Verification items for the finished model (mm, model axes). Face numbers are marked on the shaded views. A direction names the side the tool comes from. Round coordinates to 2 decimals unless told otherwise and drop trailing zeros. Write each loop counter-clockwise with the first axis right and the second up, starting at its lowest first coordinate (ties: lowest second). Pieces come first, ordered by that corner, then holes.
from build123d import *

# Parameters (mm, degrees)
BOSS_EXTRUDE1_DEPTH = 15.85
SHELL1_T            = -1.5


with BuildPart() as part:
    # Sketch1 → Boss-Extrude1 (new body)
    with BuildSketch(Plane(origin=(0, 0, 0), x_dir=(0, 0, -1), z_dir=(1, 0, 0))):
        with BuildLine():
            Line((0, 9.5), (0, 0))
            Line((0, 0), (-7.8, 0))
            ThreePointArc((-7.8, 0), (-5.600175557, 6.145933615), (0, 9.5))
        make_face()
    extrude(amount=-BOSS_EXTRUDE1_DEPTH)

    # Shell1
    shell1_openings = [part.faces().sort_by_distance(p)[0] for p in [
        (-7.925, 0, 3.9),
    ]]
    offset(amount=SHELL1_T, openings=shell1_openings, kind=Kind.INTERSECTION)


solid = part.part
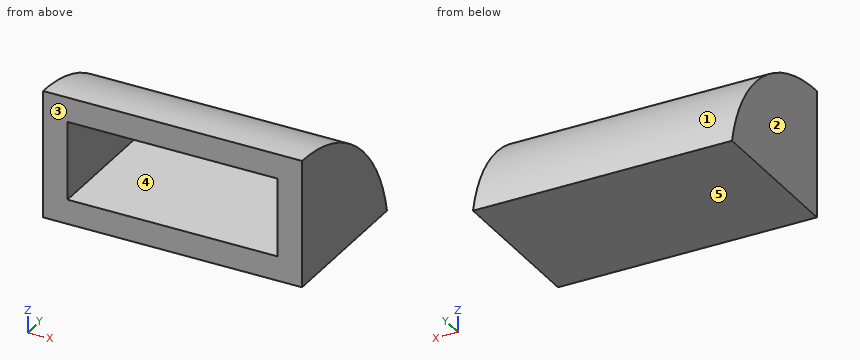
Q1. Sectioned sample at B-B (x = -2.75). Enter the section's corners in (y, z), plus the area to 3 significant figures.
Recorded:
outline: (0, 0) - (9.5, 0) arc R9.69 ccw to (0, 7.8) - (0, 6.3) arc R8.19 cw to (7.45, 1.5) - (0, 1.5) - close
area: 29.8 mm2
Q2. Tool access check on the marked faces 4 and 5. Record the directions out of +Z, -Z, +X, -X, +Y, -Y that give a thin tool (end or side, any length) a straight path to the whole face; none if there is none.
Recorded:
face 4: -Y
face 5: -Z, +X, -X, +Y, -Y
Q3. Sectioned sample at D-D (y = 1.5). Enter the section's corners in (x, z).
Recorded:
outline: (-15.85, 0) - (0, 0) - (0, 7.68) - (-15.85, 7.68) - close; hole (-14.35, 1.5) - (-1.5, 1.5) - (-1.5, 6.16) - (-14.35, 6.16) - close
Q4. Sectioned sample at C-C (z = 5). Enter the section's corners in (x, y).
Recorded:
outline: (-15.85, 0) - (-14.35, 0) - (-14.35, 4.43) - (-1.5, 4.43) - (-1.5, 0) - (0, 0) - (0, 6.81) - (-15.85, 6.81) - close
Q5. Material ranges on line 1 along X through (y, z) = (5.25, 2.25); line 2 along Z through (x, y) = (-7.75, 5.25); line 3 along Z through (x, y) = (-10.25, 3.25), recorded low to high.
Recorded:
line 1: x = -15.85 to -14.35, -1.5 to 0
line 2: z = 0 to 1.5, 4.39 to 6.25
line 3: z = 0 to 1.5, 5.63 to 7.24
Q6. Release check for a two-part mould opening along Y. For the marked faces 1, 2 and 3 record: released by +Y, released by -Y, zero draft, split by the parting line, or undercut.
Recorded:
face 1: released by +Y
face 2: zero draft
face 3: released by -Y
Q7. Sectioned sample at A-A (y = 6.25). Enter the section's corners in (x, z), plus the area to 3 significant figures.
Recorded:
outline: (-15.85, 0) - (0, 0) - (0, 5.51) - (-15.85, 5.51) - close; hole (-14.35, 1.5) - (-1.5, 1.5) - (-1.5, 3.4) - (-14.35, 3.4) - close
area: 63.0 mm2
Q8. Depth check by flat-ended pin: P1, Ø3, axis at x = -12.5, y = 7, coming from the +Z side; P2, Ø4, axis at x = -5.5, z = 4.5, coming from the +Y side. Enter the tip coordinate at first touch or a pass-through.
Recorded:
P1: stops at z = 6.09
P2: stops at y = 8.64
